Verification items for the finished model (mm, model axes). Face numbers are marked on the shaded views. A direction names the side the tool comes from. Give positions to 0.01 mm unless a question says otherwise; leave off trailing zeros. Write each loop counter-clockwise with the first axis right and the second up, starting at its lowest first coordinate (ties: lowest second). Pieces come first, ordered by that corner, then holes.
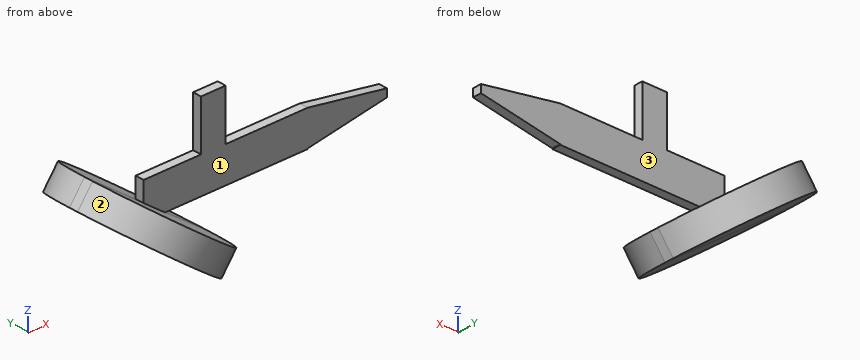
from build123d import *

# Parameters (mm, degrees)
BOSS_EXTRUDE2_DEPTH = 4
SKETCH2_W           = 66.649543755
SKETCH2_H           = 4
BOSS_EXTRUDE3_DEPTH = 11.554247081
CUT_EXTRUDE1_DEPTH  = 15


with BuildPart() as part:
    # Sketch1 → Boss-Extrude2 (new body)
    with BuildSketch(Plane(origin=(0, 0, 0), x_dir=(1, 0, 0), z_dir=(0, 1, 0))):
        Polygon((-62.077281721, 8.137219556), (-55.223313467, -1.164594503), (-31.821995465, 16.078481919), (-31.821995465, 7.098752834), (-5.630045351, 7.098752834), (-5.630045351, -15.176643991), (5.630045351, -15.176643991), (5.630045351, 7.098752834), (5.630045351, 7.343537415), (43.082086168, 7.343537415), (89.835941043, 7.343537415), (89.835941043, 23.009750567), (43.082086168, 23.009750567), (43.082086168, 23.254535147), (-22.083066084, 23.254535147), (-1.566709209, 38.371850739), (-8.420677463, 47.673664798), align=None)
    extrude(amount=-BOSS_EXTRUDE2_DEPTH)

    # Sketch2 → Boss-Extrude3 (add)
    with BuildSketch(Plane(origin=(-25.730067539, 0, -34.919377374), x_dir=(-0.8050558373533647, 0, 0.5931990380498546), z_dir=(-0.5931990380498546, 0, -0.8050558373533647))):
        with BuildLine():
            Line((-21.500856552, 0), (45.148687203, 0))
            ThreePointArc((45.148687203, 0), (11.823915325, 31.384733348), (-21.500856552, 0))
        make_face()
        with Locations((11.823915325, -2)):
            Rectangle(SKETCH2_W, SKETCH2_H)
        with BuildLine():
            ThreePointArc((-21.500856552, -4), (11.823915325, -35.384733348), (45.148687203, -4))
            Line((45.148687203, -4), (-21.500856552, -4))
        make_face()
    extrude(amount=-BOSS_EXTRUDE3_DEPTH)

    # Sketch3 → Cut-Extrude1 (cut)
    with BuildSketch(Plane.XZ.offset(4)):
        Polygon((79.345991619, -13.419165553), (79.345991619, -16.934122428), (43.082086168, -23.009750567), (79.345991619, -23.009750567), (89.835941043, -23.009750567), (89.835941043, -7.343537415), (79.345991619, -7.343537415), (43.082086168, -7.343537415), align=None)
    extrude(amount=-CUT_EXTRUDE1_DEPTH, mode=Mode.SUBTRACT)


solid = part.part
Item 1: Set-up check for the marked faces 1, 2 and 3: record each of +Z, -Z, +X, -X, +Y, -Y from which the full face is reachable in a straight line by a thin tool's end or side.
Answer key:
face 1: +Z, +X, -Y
face 2: -Y
face 3: +Z, +X, +Y
Item 2: Sectioned sample at B-B on z = 11. Record the cut outline in (x, y), then the cut area to 3 significant figures.
Answer key:
outline: (-5.63, -4) - (5.63, -4) - (5.63, 0) - (-5.63, 0) - close
area: 45.0 mm2
Item 3: Depth check by flat-ended pin: pin 1 (6 mm diameter, centred on y = 2, z = -28, fed in from -X); pin 2 (11.5 mm diameter, centred on x = 41.5, z = 2, fed in from -Y); pin 3 (2 mm diameter, centred on y = -1.5, z = 8, fed in from -X); pin 4 (2 mm diameter, centred on x = 10.5, y = -3, fed in from -Z). Enter the tip coordinate at first touch or a pass-through.
Answer key:
pin 1: stops at x = -39.19
pin 2: passes through
pin 3: stops at x = -5.63
pin 4: stops at z = -23.25
Item 4: Sectioned sample at A-A on x = 2.5. Record the cut outline in (y, z).
Answer key:
outline: (-4, -23.25) - (0, -23.25) - (0, 15.18) - (-4, 15.18) - close
Item 5: Scan lines: line 1 along Y through (x, z) = (-5, -20); line 2 along X through (y, z) = (-2, 11.5); line 3 along X through (y, z) = (12.5, -23). Record each from-to range of solid material in increasing order.
Answer key:
line 1: y = -4 to 0
line 2: x = -5.63 to 5.63
line 3: x = -41.91 to -22.43
